Check sheet for the modelled part. Datum: model origin and axes. Units: mm. A direction names the side the tool comes from. Give positions to 0.01 mm unless a question says otherwise; leave off trailing zeros. Loops run counter-clockwise (first coordinate to the right, second up) from the corner with the lowest first, then second, coordinate; pieces in that order, holes last. Notation, with made-up numbers: (-13.5, 86.5) -> (33.5, 86.5) arc R16 ccw to (33.5, 104.5) -> close; hole circle Ø1 at (85.5, 49). An arc over 180 degrees is marked (long way). Write each question's results on one line, items separated by ' | '. Start each with the question number.
Item 1: Mould release check, pull along X, two halves, no side actions. Record for faces 1 (the face through (8, 12.7, 13)), 2 (the face through (4.496, 0, 13)), 3 (the face through (-9.878, 7.407, 12.522)): pulls with the +X half, pulls with the -X half, needs draft (parallel to the pull), parting line crosses it, or undercut.
Item 2: Access from +Z, -Z, +X, -X, +Y, -Y to the whole of each face (thin tool, end or side, straight path). Record for faces 4 (the face through (-12.7, 5, 13)), 5 (the face through (-4.496, 0, 13)), 6 (the face through (0, 4.496, 13)), 7 (the face through (11.57, -3.24, 12.52)).
Item 3: Gauge pin test, flat ends, axial feed: pin 1 Ø1.6 at (x, z) = (-0.5, 12.5) entering from -Y; pin 2 Ø3.5 at (y, z) = (0, 12.5) entering from -X; pin 3 Ø1.6 at (x, z) = (0, 18) entering from +Y. Record the tip position at first contact, or that the pin passes through.
Item 4: Cross-section at A-A on x = 0. Enter the section's corners in (y, z).
Item 5: Scan lines: line 1 along Y through (x, z) = (0, 20.75); line 2 along X through (y, z) = (-3.75, 16); line 3 along Y through (x, z) = (-5.5, 5.5). Record each from-to range of solid material in increasing order.
Autodesk Inventor part; units mm, degrees
ref_plane "YZ Plane" through (0, 0, 0) normal (1, 0, 0) x (0, 1, 0)
ref_plane "XZ Plane" through (0, 0, 0) normal (0, 1, 0) x (-1, 0, 0)
ref_plane "XY Plane" through (0, 0, 0) normal (0, 0, 1) x (1, 0, 0)
sketch "Sketch1" plane through (0, 0, 0) normal (0, 0, 1) x (1, 0, 0)
  arc A0 (-12.6998, -10.5664) -> (-10.5664, -12.6998) centre (-10.5918, -10.5918) ccw
  arc A1 (-9.5504, -12.7) -> (-10.5664, -12.6998) centre (-10.0584, -12.7) ccw
  line L0 (-9.5504, -12.7) -> (-6.3331, -12.7)
  arc A2 (-5.3171, -12.7) -> (-6.3331, -12.7) centre (-5.8251, -12.7) ccw
  line L1 (-5.3171, -12.7) -> (-4.3434, -12.7)
  arc A3 (-4.3434, -12.7) -> (-4.3434, -10.4902) centre (-4.3434, -11.5951) ccw
  line L2 (-4.3434, -10.4902) -> (-6.4748, -10.4902)
  arc A4 (-7.1932, -8.7558) -> (-6.4748, -10.4902) centre (-6.4748, -9.4742) ccw
  line L3 (-7.1932, -8.7558) -> (-3.8632, -5.4257)
  arc A5 (-1.6181, -4.4958) -> (-3.8632, -5.4257) centre (-1.6181, -7.6708) ccw
  line L4 (-1.6181, -4.4958) -> (1.6181, -4.4958)
  arc A6 (3.8632, -5.4257) -> (1.6181, -4.4958) centre (1.6181, -7.6708) ccw
  line L5 (3.8632, -5.4257) -> (7.1932, -8.7558)
  arc A7 (6.4748, -10.4902) -> (7.1932, -8.7558) centre (6.4748, -9.4742) ccw
  line L6 (6.4748, -10.4902) -> (4.3434, -10.4902)
  arc A8 (4.3434, -10.4902) -> (4.3434, -12.7) centre (4.3434, -11.5951) ccw
  line L7 (4.3434, -12.7) -> (5.3171, -12.7)
  arc A9 (6.3331, -12.7) -> (5.3171, -12.7) centre (5.8251, -12.7) ccw
  line L8 (6.3331, -12.7) -> (9.5504, -12.7)
  arc A10 (10.5664, -12.6998) -> (9.5504, -12.7) centre (10.0584, -12.7) ccw
  arc A11 (10.5664, -12.6998) -> (12.6998, -10.5664) centre (10.5918, -10.5918) ccw
  arc A12 (12.7, -9.5504) -> (12.6998, -10.5664) centre (12.7, -10.0584) ccw
  line L9 (12.7, -9.5504) -> (12.7, -6.3331)
  arc A13 (12.7, -5.3171) -> (12.7, -6.3331) centre (12.7, -5.8251) ccw
  line L10 (12.7, -5.3171) -> (12.7, -4.3434)
  arc A14 (12.7, -4.3434) -> (10.4902, -4.3434) centre (11.5951, -4.3434) ccw
  line L11 (10.4902, -4.3434) -> (10.4902, -6.4748)
  arc A15 (8.7558, -7.1932) -> (10.4902, -6.4748) centre (9.4742, -6.4748) ccw
  line L12 (8.7558, -7.1932) -> (5.4257, -3.8632)
  arc A16 (4.4958, -1.6181) -> (5.4257, -3.8632) centre (7.6708, -1.6181) ccw
  line L13 (4.4958, -1.6181) -> (4.4958, 1.6181)
  arc A17 (5.4257, 3.8632) -> (4.4958, 1.6181) centre (7.6708, 1.6181) ccw
  line L14 (5.4257, 3.8632) -> (8.7558, 7.1932)
  arc A18 (10.4902, 6.4748) -> (8.7558, 7.1932) centre (9.4742, 6.4748) ccw
  line L15 (10.4902, 6.4748) -> (10.4902, 4.3434)
  arc A19 (10.4902, 4.3434) -> (12.7, 4.3434) centre (11.5951, 4.3434) ccw
  line L16 (12.7, 4.3434) -> (12.7, 5.3171)
  arc A20 (12.7, 6.3331) -> (12.7, 5.3171) centre (12.7, 5.8251) ccw
  line L17 (12.7, 6.3331) -> (12.7, 9.5504)
  arc A21 (12.6998, 10.5664) -> (12.7, 9.5504) centre (12.7, 10.0584) ccw
  arc A22 (12.6998, 10.5664) -> (10.5664, 12.6998) centre (10.5918, 10.5918) ccw
  arc A23 (9.5504, 12.7) -> (10.5664, 12.6998) centre (10.0584, 12.7) ccw
  line L18 (9.5504, 12.7) -> (6.3331, 12.7)
  arc A24 (5.3171, 12.7) -> (6.3331, 12.7) centre (5.8251, 12.7) ccw
  line L19 (5.3171, 12.7) -> (4.3434, 12.7)
  arc A25 (4.3434, 12.7) -> (4.3434, 10.4902) centre (4.3434, 11.5951) ccw
  line L20 (4.3434, 10.4902) -> (6.4748, 10.4902)
  arc A26 (7.1932, 8.7558) -> (6.4748, 10.4902) centre (6.4748, 9.4742) ccw
  line L21 (7.1932, 8.7558) -> (3.8632, 5.4257)
  arc A27 (1.6181, 4.4958) -> (3.8632, 5.4257) centre (1.6181, 7.6708) ccw
  line L22 (1.6181, 4.4958) -> (-1.6181, 4.4958)
  arc A28 (-3.8632, 5.4257) -> (-1.6181, 4.4958) centre (-1.6181, 7.6708) ccw
  line L23 (-3.8632, 5.4257) -> (-7.1932, 8.7558)
  arc A29 (-6.4748, 10.4902) -> (-7.1932, 8.7558) centre (-6.4748, 9.4742) ccw
  line L24 (-6.4748, 10.4902) -> (-4.3434, 10.4902)
  arc A30 (-4.3434, 10.4902) -> (-4.3434, 12.7) centre (-4.3434, 11.5951) ccw
  line L25 (-4.3434, 12.7) -> (-5.3171, 12.7)
  arc A31 (-6.3331, 12.7) -> (-5.3171, 12.7) centre (-5.8251, 12.7) ccw
  line L26 (-6.3331, 12.7) -> (-9.5504, 12.7)
  arc A32 (-10.5664, 12.6998) -> (-9.5504, 12.7) centre (-10.0584, 12.7) ccw
  arc A33 (-10.5664, 12.6998) -> (-12.6998, 10.5664) centre (-10.5918, 10.5918) ccw
  arc A34 (-12.7, 9.5504) -> (-12.6998, 10.5664) centre (-12.7, 10.0584) ccw
  line L27 (-12.7, 9.5504) -> (-12.7, 6.3331)
  arc A35 (-12.7, 5.3171) -> (-12.7, 6.3331) centre (-12.7, 5.8251) ccw
  line L28 (-12.7, 5.3171) -> (-12.7, 4.3434)
  arc A36 (-12.7, 4.3434) -> (-10.4902, 4.3434) centre (-11.5951, 4.3434) ccw
  line L29 (-10.4902, 4.3434) -> (-10.4902, 6.4748)
  arc A37 (-8.7558, 7.1932) -> (-10.4902, 6.4748) centre (-9.4742, 6.4748) ccw
  line L30 (-8.7558, 7.1932) -> (-5.4257, 3.8632)
  arc A38 (-4.4958, 1.6181) -> (-5.4257, 3.8632) centre (-7.6708, 1.6181) ccw
  line L31 (-4.4958, 1.6181) -> (-4.4958, -1.6181)
  arc A39 (-5.4257, -3.8632) -> (-4.4958, -1.6181) centre (-7.6708, -1.6181) ccw
  line L32 (-5.4257, -3.8632) -> (-8.7558, -7.1932)
  arc A40 (-10.4902, -6.4748) -> (-8.7558, -7.1932) centre (-9.4742, -6.4748) ccw
  line L33 (-10.4902, -6.4748) -> (-10.4902, -4.3434)
  arc A41 (-10.4902, -4.3434) -> (-12.7, -4.3434) centre (-11.5951, -4.3434) ccw
  line L34 (-12.7, -4.3434) -> (-12.7, -5.3171)
  arc A42 (-12.7, -6.3331) -> (-12.7, -5.3171) centre (-12.7, -5.8251) ccw
  line L35 (-12.7, -6.3331) -> (-12.7, -9.5504)
  arc A43 (-12.6998, -10.5664) -> (-12.7, -9.5504) centre (-12.7, -10.0584) ccw
  circle A44 centre (0, 0) radius 2.6035
extrude "Extrusion1" add sketch "Sketch1" along normal blind 25.4
properties part number "1010-3.125-CL"
Answer sheet:
1) face 1: needs draft | face 2: pulls with the +X half | face 3: undercut
2) face 4: +Z, -Z, -X, +Y, -Y | face 5: +Z, -Z, -X | face 6: +Z, -Z, +Y | face 7: +Z, -Z
3) pin 1: stops at y = -4.5 | pin 2: stops at x = -4.5 | pin 3: stops at y = 4.5
4) outline: (-4.5, 0) -> (-2.6, 0) -> (-2.6, 25.4) -> (-4.5, 25.4) -> close; (2.6, 0) -> (4.5, 0) -> (4.5, 25.4) -> (2.6, 25.4) -> close
5) line 1: y = -4.5 to -2.6, 2.6 to 4.5 | line 2: x = -12.53 to -10.66, -5.32 to 5.32, 10.66 to 12.53 | line 3: y = -12.31 to -10.49, -7.06 to -3.94, 3.94 to 7.06, 10.49 to 12.31
